The listing builds one solid part. Answer for the finished solid, in the listing's coordinates (mm). A direction names the side the tool comes from. Round coordinates to 2 decimals unless told otherwise and drop trailing zeros. Write each loop counter-clockwise with the first axis right and the second up, starting at its lowest first coordinate (ties: lowest second). Pieces come first, ordered by that corner, then holes.
from build123d import *

# Parameters (mm, degrees)
BOX003_W          = 35.6
BOX003_H          = 19
BOX003_DEPTH      = 0.2
CYLINDER003_R     = 1.5
CYLINDER003_DEPTH = 10
CYLINDER004_R     = 1.5
CYLINDER004_DEPTH = 10
CYLINDER005_R     = 1.5
CYLINDER005_DEPTH = 10
CYLINDER006_R     = 1.5
CYLINDER006_DEPTH = 10
BOX001_W          = 35.6
BOX001_H          = 33.5
BOX001_DEPTH      = 1.6
BOX002_W          = 35.6
BOX002_H          = 23
BOX002_DEPTH      = 1.6


with BuildPart() as cube001:
    # Box003 → Box003 (new body)
    with BuildSketch(Plane(origin=(0, 9, 53.2), x_dir=(1, 0, 0), z_dir=(0, 0, 1))):
        with Locations((17.8, 9.5)):
            Rectangle(BOX003_W, BOX003_H)
    extrude(amount=BOX003_DEPTH)


with BuildPart() as cylinder003:
    # Cylinder003 → Cylinder003 (new body)
    with BuildSketch(Plane(origin=(2.5, 2.5, 45), x_dir=(1, 0, 0), z_dir=(0, 0, 1))):
        Circle(CYLINDER003_R)
    extrude(amount=CYLINDER003_DEPTH)


with BuildPart() as cylinder004:
    # Cylinder004 → Cylinder004 (new body)
    with BuildSketch(Plane(origin=(33.5, 2.5, 45), x_dir=(1, 0, 0), z_dir=(0, 0, 1))):
        Circle(CYLINDER004_R)
    extrude(amount=CYLINDER004_DEPTH)


with BuildPart() as cylinder005:
    # Cylinder005 → Cylinder005 (new body)
    with BuildSketch(Plane(origin=(2.5, 31, 45), x_dir=(1, 0, 0), z_dir=(0, 0, 1))):
        Circle(CYLINDER005_R)
    extrude(amount=CYLINDER005_DEPTH)


with BuildPart() as fusion017:
    # Cylinder006 → Cylinder006 (new body)
    with BuildSketch(Plane(origin=(33.5, 31, 45), x_dir=(1, 0, 0), z_dir=(0, 0, 1))):
        Circle(CYLINDER006_R)
    extrude(amount=CYLINDER006_DEPTH)

    # Fusion017: union Cylinder003, Cylinder004, Cylinder005
    add(cylinder003.part)
    add(cylinder004.part)
    add(cylinder005.part)


with BuildPart() as cut:
    # Box001 → Box001 (new body)
    with BuildSketch(Plane.XY.offset(50)):
        with Locations((17.8, 16.75)):
            Rectangle(BOX001_W, BOX001_H)
    extrude(amount=BOX001_DEPTH)

    # Cut: cut Fusion017
    add(fusion017.part, mode=Mode.SUBTRACT)


with BuildPart() as oled001:
    # Box002 → Box002 (new body)
    with BuildSketch(Plane(origin=(0, 5, 51.6), x_dir=(1, 0, 0), z_dir=(0, 0, 1))):
        with Locations((17.8, 11.5)):
            Rectangle(BOX002_W, BOX002_H)
    extrude(amount=BOX002_DEPTH)

    # Fusion018: union Cube001, Cut
    add(cube001.part)
    add(cut.part)


solid = oled001.part
1. Section B-B on z = 50.45 is taken. Determine the outline of the cut face in (x, y).
Geometry says:
outline: (0, 0) - (35.6, 0) - (35.6, 33.5) - (0, 33.5) - close; hole circle Ø3 at (2.5, 2.5); hole circle Ø3 at (2.5, 31); hole circle Ø3 at (33.5, 2.5); hole circle Ø3 at (33.5, 31)
2. Section D-D on y = 7 is taken. Determine the outline of the cut face in (x, z).
Geometry says:
outline: (0, 50) - (35.6, 50) - (35.6, 53.2) - (0, 53.2) - close
3. A tool of negligible diameter and unlimited length cuts with its end or side. For faces 4 (the face through (18, 7, 53.2)), 5 (the face through (32.3, 1.6, 50.8)), 6 (the face through (18, 28, 52)), from which of +Z, -Z, +X, -X, +Y, -Y can it reach the whole face along a straight path? Write none if from no direction.
Geometry says:
face 4: +Z, +X, -X, -Y
face 5: +Z, -Z
face 6: +Z, +X, -X, +Y
4. Given pin 1 (2.5 mm diameter, centred on x = 16.5, y = 1.5, fed in from +Z); pin 2 (1.8 mm diameter, centred on x = 33.5, y = 31, fed in from +Z); pin 3 (1.2 mm diameter, centred on x = 26.5, y = 7, fed in from +Z); pin 4 (1.3 mm diameter, centred on x = 18.5, z = 53, fed in from -Y), each flat-ended and moving along its own axis, determine where each tip first touches the part or whether it passes through.
Geometry says:
pin 1: stops at z = 51.6
pin 2: passes through
pin 3: stops at z = 53.2
pin 4: stops at y = 5
5. For a pull along X with two mould halves and no side action, classify faces 1 (the face through (2.175, 1.036, 50.789)), 2 (the face through (18, 19, 53.4)), 3 (the face through (35.6, 17, 52)) as released by +X, released by -X, zero draft, split by the parting line, or undercut.
Geometry says:
face 1: undercut
face 2: zero draft
face 3: released by +X
6. Section A-A on y = 31 is taken. Determine the outline of the cut face in (x, z), plus the area to 3 significant figures.
Geometry says:
outline: (0, 50) - (1, 50) - (1, 51.6) - (0, 51.6) - close; (4, 50) - (32, 50) - (32, 51.6) - (4, 51.6) - close; (35, 50) - (35.6, 50) - (35.6, 51.6) - (35, 51.6) - close
area: 47.4 mm2
7. Section C-C on x = 29 is taken. Determine the outline of the cut face in (y, z), plus the area to 3 significant figures.
Geometry says:
outline: (0, 50) - (33.5, 50) - (33.5, 51.6) - (28, 51.6) - (28, 53.4) - (9, 53.4) - (9, 53.2) - (5, 53.2) - (5, 51.6) - (0, 51.6) - close
area: 94.2 mm2
8. Straight lines are drawn through the part: line 1 along X through (y, z) = (2.5, 50.7); line 2 along Y through (x, z) = (2.5, 51); line 3 along X through (y, z) = (30.5, 51.1). For each, find the intervals that lie inside material, in ascending order.
Geometry says:
line 1: x = 0 to 1, 4 to 32, 35 to 35.6
line 2: y = 0 to 1, 4 to 29.5, 32.5 to 33.5
line 3: x = 0 to 1.09, 3.91 to 32.09, 34.91 to 35.6
